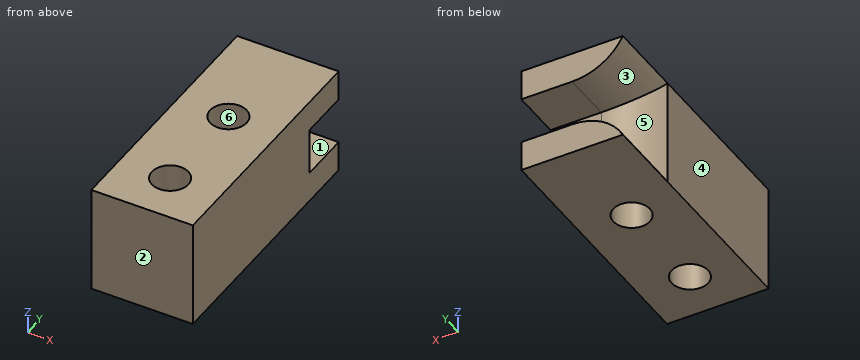
from build123d import *

# Parameters (mm, degrees)
SKETCH1_W                       = 10
SKETCH1_H                       = 10.6
BOSS_EXTRUDE1_DEPTH             = 20
CUT_EXTRUDE1_DEPTH              = 25.745908753
BOSS_EXTRUDE2_DEPTH             = 5
BOSS_EXTRUDE2_DIRECTION_2_REACH = 26.746
SKETCH5_R                       = 1.8
CUT_EXTRUDE2_DEPTH              = 29.937173447


with BuildPart() as part:
    # Sketch1 → Boss-Extrude1 (new body)
    with BuildSketch(Plane(origin=(0, 0, 0), x_dir=(1, 0, 0), z_dir=(0, 1, 0))):
        with Locations((5, 5.3)):
            Rectangle(SKETCH1_W, SKETCH1_H)
    extrude(amount=BOSS_EXTRUDE1_DEPTH)

    # Sketch3 → Cut-Extrude1 (cut, through all)
    with BuildSketch(Plane.XY):
        with BuildLine():
            Line((0, 17.31662479), (0, 20))
            Line((0, 20), (5, 20))
            ThreePointArc((5, 20), (2.162725669, 19.286764074), (0, 17.31662479))
        make_face()
    extrude(amount=-CUT_EXTRUDE1_DEPTH, mode=Mode.SUBTRACT)

    # Sketch4 → Boss-Extrude2 (add)
    with BuildSketch(Plane(origin=(0, 20, 0), x_dir=(1, 0, 0), z_dir=(0, 1, 0))):
        with BuildLine():
            Line((10, 10.6), (0, 10.6))
            ThreePointArc((0, 10.6), (2.084524053, 8.407540088), (5, 7.6))
            Line((5, 7.6), (10, 7.6))
            Line((10, 7.6), (10, 10.6))
        make_face()
        with BuildLine():
            Line((0, 0), (10, 0))
            Line((10, 0), (10, 3))
            Line((10, 3), (5, 3))
            ThreePointArc((5, 3), (2.084524053, 2.192459912), (0, 0))
        make_face()
    extrude(amount=BOSS_EXTRUDE2_DEPTH)

    # Sketch4 → Boss-Extrude2 direction 2 (add, up to next)
    with BuildSketch(Plane(origin=(0, 20, 0), x_dir=(1, 0, 0), z_dir=(0, 1, 0)), mode=Mode.PRIVATE) as boss_extrude2_direction_2_sk1:
        with BuildLine():
            Line((10, 10.6), (0, 10.6))
            ThreePointArc((0, 10.6), (2.084524053, 8.407540088), (5, 7.6))
            Line((5, 7.6), (10, 7.6))
            Line((10, 7.6), (10, 10.6))
        make_face()
    boss_extrude2_direction_2_tool1 = extrude(boss_extrude2_direction_2_sk1.sketch, amount=-BOSS_EXTRUDE2_DIRECTION_2_REACH, mode=Mode.PRIVATE) - part.part
    # Sketch4 → Boss-Extrude2 direction 2 (add, up to next)
    with BuildSketch(Plane(origin=(0, 20, 0), x_dir=(1, 0, 0), z_dir=(0, 1, 0)), mode=Mode.PRIVATE) as boss_extrude2_direction_2_sk2:
        with BuildLine():
            Line((0, 0), (10, 0))
            Line((10, 0), (10, 3))
            Line((10, 3), (5, 3))
            ThreePointArc((5, 3), (2.084524053, 2.192459912), (0, 0))
        make_face()
    boss_extrude2_direction_2_tool2 = extrude(boss_extrude2_direction_2_sk2.sketch, amount=-BOSS_EXTRUDE2_DIRECTION_2_REACH, mode=Mode.PRIVATE) - part.part
    add(boss_extrude2_direction_2_tool1.solids().sort_by_distance((5.642353, 20, -9.211407))[0])
    add(boss_extrude2_direction_2_tool2.solids().sort_by_distance((5.642353, 20, -1.388593))[0])

    # Sketch5 → Cut-Extrude2 (cut, through all)
    with BuildSketch(Plane.XY):
        with Locations((5, 14.8)):
            Circle(SKETCH5_R)
        with Locations((5, 4.8)):
            Circle(SKETCH5_R)
    extrude(amount=-CUT_EXTRUDE2_DEPTH, mode=Mode.SUBTRACT)


solid = part.part
Geometry: final body of the model. Coordinates: model frame, mm. Face numbers are marked on the shaded views. A direction names the side the tool comes from. Give positions to 0.01 mm unless a question says otherwise; leave off trailing zeros. Write each loop counter-clockwise with the first axis right and the second up, starting at its lowest first coordinate (ties: lowest second). Pieces come first, ordered by that corner, then holes.
(1) Ray query, line 1 (Y direction, x = 5, z = -7.5); line 2 (Y direction, x = 5, z = -7.75); line 3 (X direction, y = 3.75, z = -7.5). Return the intervals inside material, ascending.
(2) Cut plane D-D, the plane y = 23. Return loops of the section in (x, z), then the cut area to 3 significant figures.
(3) Cut plane B-B, the plane y = 4.8. Return loops of the section in (x, z), then the cut area to 3 significant figures.
(4) Cut plane A-A, the plane z = -7. Return loops of the section in (x, y).
(5) Mould query, pull axis Y, two halves, no side actions, for the marked faces 4, 5 and 6. Classes: released by +Y, released by -Y, zero draft, split by the parting line, or undercut.
(6) Cut plane C-C, the plane x = 7.25. Return loops of the section in (y, z), then the cut area to 3 significant figures.
(7) First-contact query: P1, Ø2.5, axis at x = 8, z = -5.5, coming from the +Y side; P2, Ø3, axis at x = 5, y = 4.8, coming from the +Z side. Flat tips, straight axial feed; report the tip coordinate or a pass-through.
(8) Access query for the marked faces 1, 2 and 3. Directions: +Z, -Z, +X, -X, +Y, -Y. A direction counts if a zero-diameter tool reaches every point of the face in a straight line with its end or side. Return the directions, or none.
Values follow:
1. line 1: y = 0 to 3, 6.6 to 13, 16.6 to 20
1. line 2: y = 0 to 3, 6.6 to 13, 16.6 to 25
1. line 3: x = 0 to 3.54, 6.46 to 10
2. outline: (0, -10.6) - (10, -10.6) - (10, -7.6) - (5, -7.6) arc R5.67 ccw to start; (0, 0) arc R5.67 ccw to (5, -3) - (10, -3) - (10, 0) - close
2. area: 51.4 mm2
3. outline: (0, -10.6) - (3.2, -10.6) - (3.2, 0) - (0, 0) - close; (6.8, -10.6) - (10, -10.6) - (10, 0) - (6.8, 0) - close
3. area: 67.8 mm2
4. outline: (0, 0) - (10, 0) - (10, 20) - (5, 20) arc R6 ccw to (0, 17.32) - close; hole circle Ø3.6 at (5, 4.8); hole circle Ø3.6 at (5, 14.8)
5. face 4: zero draft
5. face 5: released by +Y
5. face 6: undercut
6. outline: (0, -10.6) - (25, -10.6) - (25, -7.6) - (20, -7.6) - (20, -3) - (25, -3) - (25, 0) - (0, 0) - close
6. area: 242 mm2
7. P1: stops at y = 20
7. P2: passes through
8. face 1: +X, -X, +Y
8. face 2: +Z, -Z, +X, -X, -Y
8. face 3: -X, +Y
